For this review, use the dimensioned drawing (mm, ordinates from the lowest corner) and the shaded views. Give positions to 0.01 mm unless a question says otherwise; leave off trailing zeros. Order: outer loops, then holes, each group sorted by start corner. A loop starts at its lowest first (then second) coordinate and runs counter-clockwise, first axis right, second up. Notation, with made-up numbers: (-10.75, -20) -> (-6.75, -20) arc R27 ccw to (-6.75, 9) -> close; hole circle Ø6 at (59.5, 35). An arc over 180 degrees is marked (long way). Return JSON: item names as keys, results as strings.
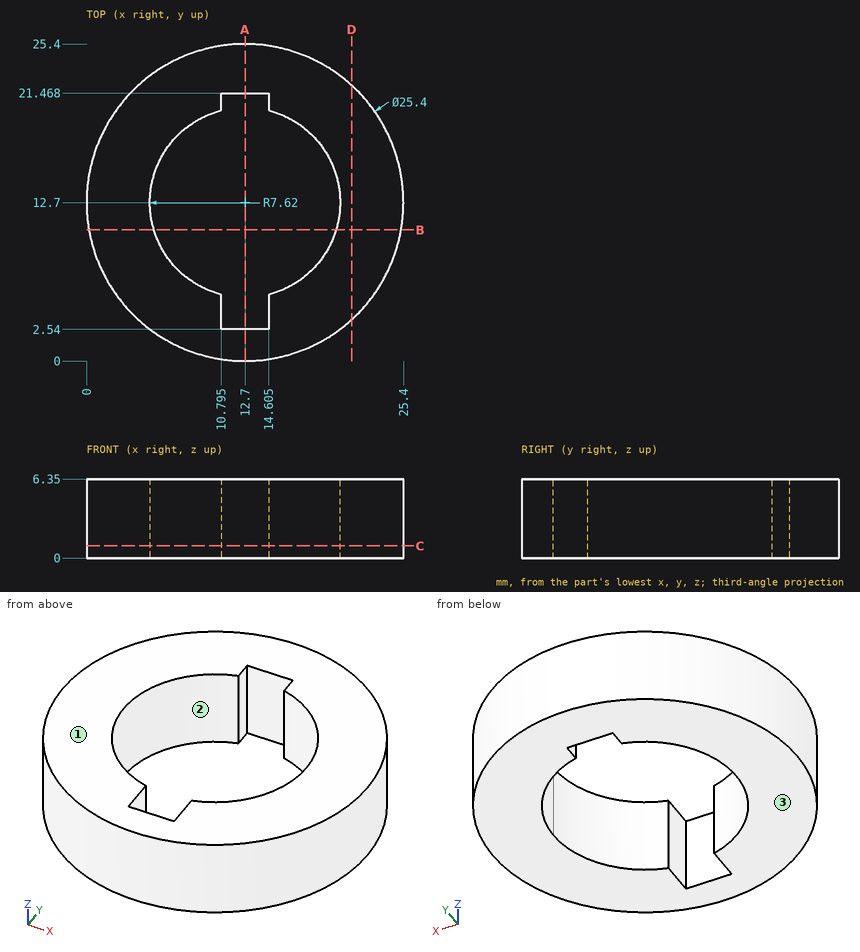
Item 1: Add section A-A (x = 12.7). Give the boundary of the cut face in (y, z), plus the area to 3 significant figures.
Result set:
{"outline": "(0, 0) -> (2.54, 0) -> (2.54, 6.35) -> (0, 6.35) -> close; (21.47, 0) -> (25.4, 0) -> (25.4, 6.35) -> (21.47, 6.35) -> close", "area": "41.1 mm^2"}
Item 2: Add section C-C (z = 1). Give the boundary of the cut face in (x, y) (3 decimals).
Result set:
{"outline": "circle Ø25.4 at (12.7, 12.7); hole (10.795, 2.54) -> (14.605, 2.54) -> (14.605, 5.322) arc R7.62 ccw to (14.605, 20.078) -> (14.605, 21.468) -> (10.795, 21.468) -> (10.795, 20.078) arc R7.62 ccw to (10.795, 5.322) -> close"}
Item 3: For pin 1 (2 mm diameter, centred on x = 10.5, z = 3.5, fed in from +Y); pin 2 (3 mm diameter, centred on y = 3.5, z = 1.5, fed in from +X); pin 3 (1.5 mm diameter, centred on x = 18, z = 3, fed in from +Y), all flat-tipped, find the tip position at first contact; note any pin that passes through.
Result set:
{"pin 1": "stops at y = 25.34", "pin 2": "stops at x = 22.8", "pin 3": "stops at y = 24.56"}
Item 4: Add section B-B (y = 10.5). Give the boundary of the cut face in (x, z), plus the area to 3 significant figures.
Result set:
{"outline": "(0.19, 0) -> (5.4, 0) -> (5.4, 6.35) -> (0.19, 6.35) -> close; (20, 0) -> (25.21, 0) -> (25.21, 6.35) -> (20, 6.35) -> close", "area": "66.2 mm^2"}
Item 5: Add section D-D (x = 21.25). Give the boundary of the cut face in (y, z), plus the area to 3 significant figures.
Result set:
{"outline": "(3.31, 0) -> (22.09, 0) -> (22.09, 6.35) -> (3.31, 6.35) -> close", "area": "119 mm^2"}
Item 6: Wall thickness on L1, parallel to X at y = 12.5, z = 3; L2, parallel to X at y = 18, z = 2 (1 decimal); L3, parallel to Y at x = 7, z = 6: over which ranges is each line inside the solid? List them lowest first. Write a range as [from, to].
Result set:
{"L1": "x = [0, 5.08], [20.32, 25.4]", "L2": "x = [1.2, 7.2], [18.2, 24.2]", "L3": "y = [1.35, 7.64], [17.76, 24.05]"}
Item 7: Mouldability with a two-part tool opening along Z and no side actions: class the marked faces 1, 2 and 3 as released by +Z, released by -Z, zero draft, split by the parting line, or undercut.
Result set:
{"face 1": "released by +Z", "face 2": "zero draft", "face 3": "released by -Z"}
